from build123d import *

# Parameters (mm, degrees)
SKETCH1_R           = 0.5
SKETCH1_R_2         = 2.07
BOSS_EXTRUDE1_DEPTH = 1.5
FILLET1_R           = 3
CHAMFER1_SIZE       = 15
FILLET2_R           = 3


with BuildPart() as part:
    # Sketch1 → Boss-Extrude1 (new, symmetric)
    with BuildSketch(Plane.XY):
        Polygon((0, 0), (50.8, 0), (50.8, 38.1), (-44.45, 38.1), (-44.45, -38.1), (0, -38.1), align=None)
        with Locations((-22.225, 19.05)):
            Circle(SKETCH1_R, mode=Mode.SUBTRACT)
        with Locations((44.45, 31.75)):
            Circle(SKETCH1_R_2, mode=Mode.SUBTRACT)
        with Locations((31.75, 31.75)):
            Circle(SKETCH1_R_2, mode=Mode.SUBTRACT)
        with Locations((19.05, 31.75)):
            Circle(SKETCH1_R_2, mode=Mode.SUBTRACT)
        with Locations((6.35, 31.75)):
            Circle(SKETCH1_R_2, mode=Mode.SUBTRACT)
        with Locations(Location((6.35, 6.35, 0), (0, 0, 180))):
            Circle(SKETCH1_R_2, mode=Mode.SUBTRACT)
        with Locations(Location((19.05, 6.35, 0), (0, 0, 180))):
            Circle(SKETCH1_R_2, mode=Mode.SUBTRACT)
        with Locations(Location((31.75, 6.35, 0), (0, 0, 180))):
            Circle(SKETCH1_R_2, mode=Mode.SUBTRACT)
        with Locations(Location((44.45, 6.35, 0), (0, 0, 180))):
            Circle(SKETCH1_R_2, mode=Mode.SUBTRACT)
        with Locations((25.4, 19.05)):
            Circle(SKETCH1_R_2, mode=Mode.SUBTRACT)
        with Locations((38.1, 19.05)):
            Circle(SKETCH1_R_2, mode=Mode.SUBTRACT)
        with Locations(Location((12.7, 19.05, 0), (0, 0, 180))):
            Circle(SKETCH1_R_2, mode=Mode.SUBTRACT)
        with Locations((-34.925, -25.4)):
            Circle(SKETCH1_R_2, mode=Mode.SUBTRACT)
        with Locations((-9.525, -25.4)):
            Circle(SKETCH1_R_2, mode=Mode.SUBTRACT)
        with Locations((-34.925, -12.7)):
            Circle(SKETCH1_R_2, mode=Mode.SUBTRACT)
        with Locations((-9.525, -12.7)):
            Circle(SKETCH1_R_2, mode=Mode.SUBTRACT)
        with Locations((-34.925, 0)):
            Circle(SKETCH1_R_2, mode=Mode.SUBTRACT)
        with Locations((-9.525, 0)):
            Circle(SKETCH1_R_2, mode=Mode.SUBTRACT)
        with Locations((-34.925, 12.7)):
            Circle(SKETCH1_R_2, mode=Mode.SUBTRACT)
        with Locations((-9.525, 12.7)):
            Circle(SKETCH1_R_2, mode=Mode.SUBTRACT)
        with Locations((-34.925, 25.4)):
            Circle(SKETCH1_R_2, mode=Mode.SUBTRACT)
        with Locations((-9.525, 25.4)):
            Circle(SKETCH1_R_2, mode=Mode.SUBTRACT)
    extrude(amount=BOSS_EXTRUDE1_DEPTH, both=True)

    # Fillet1
    fillet1_edges = [part.edges().sort_by_distance(p)[0] for p in [
        (0, -38.1, 0),
        (-44.45, -38.1, 0),
        (-44.45, 38.1, 0),
        (50.8, 38.1, 0),
        (50.8, 0, 0),
    ]]
    fillet(fillet1_edges, radius=FILLET1_R)

    # Chamfer1
    chamfer1_edges = [part.edges().sort_by_distance(p)[0] for p in [
        (0, 0, 0),
    ]]
    chamfer(chamfer1_edges, length=CHAMFER1_SIZE)

    # Fillet2
    fillet2_edges = [part.edges().sort_by_distance(p)[0] for p in [
        (15, 0, 0),
        (0, -15, 0),
    ]]
    fillet(fillet2_edges, radius=FILLET2_R)


solid = part.part
Read the model definition and answer for the solid it produces. Units are mm, in the model's axes. A direction names the side the tool comes from. Give positions to 0.01 mm unless a question says otherwise; leave off trailing zeros. Write each loop counter-clockwise with the first axis right and the second up, starting at its lowest first coordinate (ties: lowest second). Pieces come first, ordered by that corner, then holes. Notation, with made-up numbers: M -39,14 L -33,14 A15 cw -33,18 Z; hole C 34,28 d5. An arc over 180 degrees is marked long. One line per item, written item: value. Start each with the question number.
(1) Find section C-C (x = 25.4). Determine the outline of the cut face in (y, z), plus the area to 3 significant figures.
(2) A tool of negligible diameter and unlimited length cuts with its end or side. For faces 1 (the flat face through (32, 0, 0)), 2 (the cylindrical face through (-8.412, 14.445, -0.021)), from which of +Z, -Z, +X, -X, +Y, -Y can it reach the whole face along a straight path? Write none if from no direction.
(3) Find section B-B (y = 25.4). Determine the outline of the cut face in (x, z) (3 decimals).
(4) Flat-ended cylindrical pins translate along their axes: pin 1 Ø1.5 at (x, z) = (28, -1) entering from -Y; pin 2 Ø6.5 at (x, y) = (-9.525, -25.4) entering from +Z; pin 3 Ø2.5 at (x, y) = (-34.925, -12.7) entering from -Z; pin 4 Ø0.9 at (y, z) = (-29, 0) entering from +X. Find the tip coordinate at first contact, or state that the pin passes through.
(5) Find section D-D (z = 0.7). Give the number of separate pieces and of enclosed holes in the cut face, plus the area to 3 significant figures.
(6) Find section A-A (x = 6.35). Determine the outline of the cut face in (y, z), plus the area to 3 significant figures.
(7) Find the intervals of material crossed by line 1 (Y direction, x = 19.05, z = 0.3); line 2 (Y direction, x = 25.4, z = 0); line 3 (X direction, y = -26.5, z = -1), in increasing order.
(8) Determine the mould class of faces 3 (the cylindrical face through (-43.55, -37.24, -0.02)), 4 (the flat face through (-8, 9, 1.5)), 5 (the cylindrical face through (36.03, 19.14, -0.02)), 6 (the cylindrical face through (49.9, 37.24, 0.02)) for opening direction X: pulls with the +X half, pulls with the -X half, needs draft (parallel to the pull), parting line crosses it, or undercut.
Results below:
1. outline: M 0,-1.5 L 16.98,-1.5 L 16.98,1.5 L 0,1.5 Z; M 21.12,-1.5 L 38.1,-1.5 L 38.1,1.5 L 21.12,1.5 Z
1. area: 102 mm^2
2. face 1: +Z, -Z, +X, -Y
2. face 2: +Z, -Z
3. outline: M -44.45,-1.5 L -36.995,-1.5 L -36.995,1.5 L -44.45,1.5 Z; M -32.855,-1.5 L -11.595,-1.5 L -11.595,1.5 L -32.855,1.5 Z; M -7.455,-1.5 L 50.8,-1.5 L 50.8,1.5 L -7.455,1.5 Z
4. pin 1: stops at y = 0
4. pin 2: stops at z = 1.5
4. pin 3: passes through
4. pin 4: stops at x = 0
5. separate pieces: 1
5. enclosed holes: 22
5. area: 5,140 mm^2
6. outline: M -8.65,-1.5 L 4.28,-1.5 L 4.28,1.5 L -8.65,1.5 Z; M 8.42,-1.5 L 29.68,-1.5 L 29.68,1.5 L 8.42,1.5 Z; M 33.82,-1.5 L 38.1,-1.5 L 38.1,1.5 L 33.82,1.5 Z
6. area: 115 mm^2
7. line 1: y = 0 to 4.28, 8.42 to 29.68, 33.82 to 38.1
7. line 2: y = 0 to 16.98, 21.12 to 38.1
7. line 3: x = -44.45 to -36.68, -33.17 to -11.28, -7.77 to 0
8. face 3: pulls with the -X half
8. face 4: needs draft
8. face 5: undercut
8. face 6: pulls with the +X half
